The model under review builds one solid part; all positions refer to its coordinate system, in mm. Give positions to 0.01 mm unless a question says otherwise; leave off trailing zeros. Order: outer loops, then holes, each group sorted by start corner. A loop starts at its lowest first (then second) coordinate and runs counter-clockwise, first axis right, second up. Notation, with made-up numbers: (-36, 46.25) -> (-3, 46.25) arc R19 cw to (-3, 63.25) -> close; hole circle Ø1 at (-39.75, 39). An arc over 180 degrees is marked (long way). Use one line per item in the form item = value.
Autodesk Inventor part; units mm, degrees
ref_plane "YZ Plane" through (0, 0, 0) normal (1, 0, 0) x (0, 1, 0)
ref_plane "XZ Plane" through (0, 0, 0) normal (0, 1, 0) x (-1, 0, 0)
ref_plane "XY Plane" through (0, 0, 0) normal (0, 0, 1) x (1, 0, 0)
sketch "Sketch1" plane through (0, 0, 0) normal (1, 0, 0) x (0, 1, 0)
  line L0 (0, 0) -> (20, 0)
  line L1 (20, 0) -> (20, 31.4)
  line L2 (20, 31.4) -> (0, 31.4)
  line L3 (0, 31.4) -> (0, 0)
  dimension "d0" = 20
  dimension "d1" = 31.4
extrude "Extrusion1" add sketch "Sketch1" along normal blind 5
fillet "Fillet1" radius 1.5875 12 edges at (0, 0, 15.7) (2.5, 0, 0) (5, 0, 15.7) (2.5, 0, 31.4) (0, 10, 31.4) (5, 10, 31.4) (2.5, 20, 31.4) (0, 20, 15.7) (5, 20, 15.7) (2.5, 20, 0) (0, 10, 0) (5, 10, 0)
sketch "Sketch2" plane through (1.5875, 1.5875, 31.4) normal (0, 0, 1) x (1, 0, 0)
  line L0 (0, 0) -> (0, 16.825)
  line L1 (1.825, 0) -> (0, 0)
  line L2 (1.825, 16.825) -> (1.825, 0)
  circle A0 centre (0.9125, 14.325) radius 0.9125
  circle A1 centre (0.9125, 12.5) radius 0.9125
  point P0 (-1.5875, -1.5875)
  dimension "d5" = 12.5
extrude "Extrusion2" add sketch "Sketch2" along normal blind 5 contours A1 | A0
properties part number "adafruit 500mAh battery"
1. For L1, parallel to Y at x = 3.55, z = 7; L2, parallel to Z at x = 1.75, y = 13.25; L3, parallel to X at y = 18.5, z = 9, list the stretches that pass through material, from the lowest coordinate up.
Values:
L1 = 0.01 to 19.99
L2 = 0 to 31.4
L3 = 0 to 5
2. The part is to be moulded in two halves that separate along Y. For faces 1 (the face through (2.51, 0.45, 0.48)), 2 (the face through (3.2, 15, 31.4)), 3 (the face through (2.51, 19.52, 0.45)), 4 (the face through (2, 10, 0)), say which applies: +Y half, -Y half, draft (parallel to the pull), parting line (faces both ways), or undercut.
Values:
face_1 = -Y half
face_2 = undercut
face_3 = +Y half
face_4 = draft
3. Add section B-B on y = 8. Give the boundary of the cut face in (x, z) (1 decimal).
Values:
outline = (0, 1.6) arc R1.6 ccw to (1.6, 0) -> (3.4, 0) arc R1.6 ccw to (5, 1.6) -> (5, 29.8) arc R1.6 ccw to (3.4, 31.4) -> (1.6, 31.4) arc R1.6 ccw to (0, 29.8) -> close
4. For pin 1 Ø2 at (x, y) = (2.5, 17.5) entering from +Z; pin 2 Ø0.9 at (x, y) = (2.5, 8) entering from +Z, all flat-tipped, find the tip position at first contact; note any pin that passes through.
Values:
pin_1 = 36.4
pin_2 = 31.4
5. Add section A-A on z = 15. Give the boundary of the cut face in (x, y) (1 decimal).
Values:
outline = (0, 1.6) arc R1.6 ccw to (1.6, 0) -> (3.4, 0) arc R1.6 ccw to (5, 1.6) -> (5, 18.4) arc R1.6 ccw to (3.4, 20) -> (1.6, 20) arc R1.6 ccw to (0, 18.4) -> close
